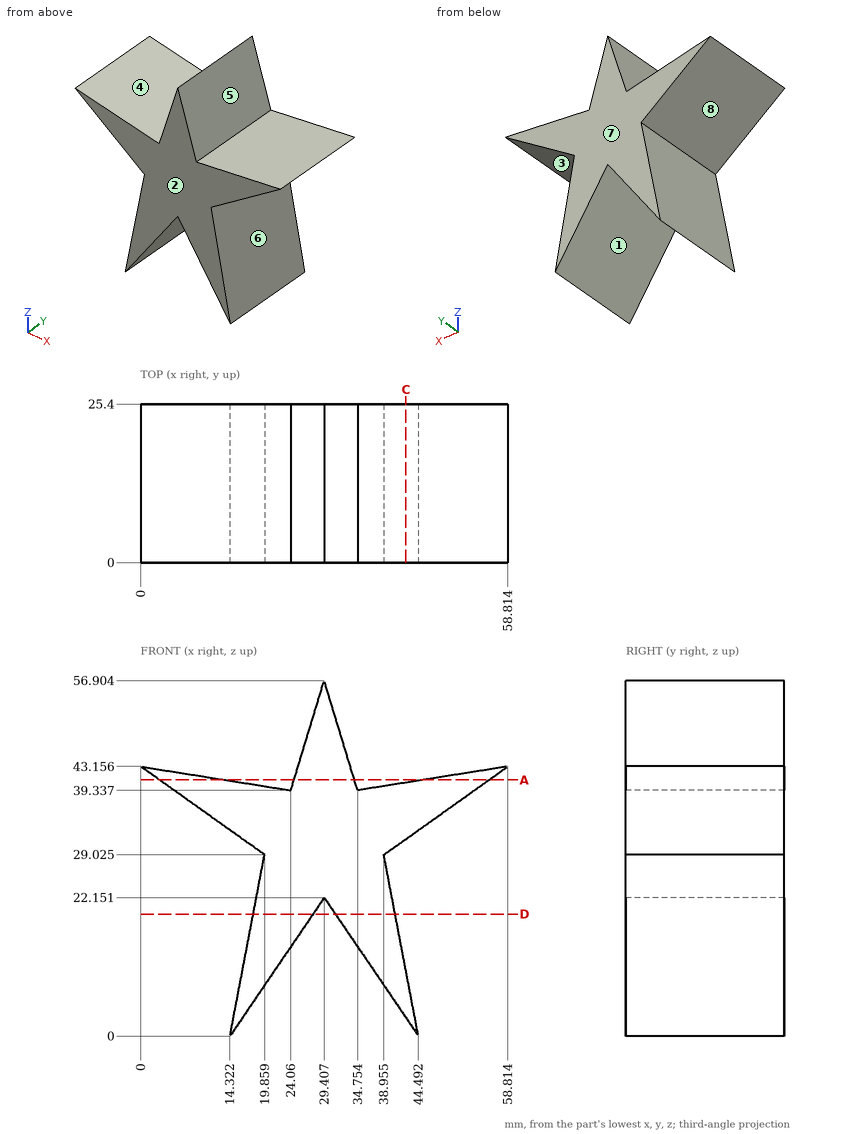
Input: dimensioned drawing with shaded views. Units: mm. Origin: part minimum x, y, z. A direction names the side the tool comes from. Coordinates: 2 decimals unless noted, no trailing zeros. Order: outer loops, then holes, each group sorted by start corner. A loop starts at its lowest first (then second) coordinate and runs counter-clockwise, first axis right, second up. Notation, with made-up numbers: (-12, 24) -> (8, 24) arc R28 cw to (8, 47) -> close; hole circle Ø10 at (36.25, 38). An arc over 180 degrees is marked (long way). Use CSV: the item, a comma, the result in double quotes.
1) Line query: line 1 (X direction, y = 24, z = 19) (1 decimal); line 2 (X direction, y = 22.5, z = 5.5) (1 decimal); line 3 (Z direction, x = 56, y = 22) (1 decimal). Output: solid intervals per line, ascending.
Findings:
line 1,"x = 17.9 to 27.3, 31.6 to 40.9"
line 2,"x = 15.4 to 18.1, 40.7 to 43.4"
line 3,"z = 41.2 to 42.7"
2) Mould query, pull axis Z, two halves, no side actions, for the marked faces 1, 2, 3 and 4. Classes: +Z half, -Z half, draft (parallel to the pull), parting line (faces both ways), or undercut.
Findings:
face 1,"-Z half"
face 2,"draft"
face 3,"undercut"
face 4,"+Z half"
3) Access query for the marked faces 5, 6, 7 and 8. Directions: +Z, -Z, +X, -X, +Y, -Y. A direction counts if a zero-diameter tool reaches every point of the face in a straight line with its end or side. Return the directions, or none.
Findings:
face 5,"+Z, +Y, -Y"
face 6,"+X, +Y, -Y"
face 7,"+Z, -Z, +X, -X, +Y"
face 8,"-X, +Y, -Y"
4) Pin query (flat end, axial travel): pin 1 Ø3 at (x, y) = (20, 2.5) entering from -Z (1 decimal); pin 2 Ø5 at (x, y) = (7.5, 18) entering from -Z; pin 3 Ø5 at (x, y) = (44, 18.5) entering from -Z; pin 4 Ø3 at (y, z) = (7, 29.5) entering from -X (1 decimal). Return the tip coordinate at first contact, or that it passes through.
Findings:
pin 1,"stops at z = 6.1"
pin 2,"stops at z = 36.04"
pin 3,"stops at z = 0"
pin 4,"stops at x = 17.1"
5) Section A-A on z = 41. Output: boundary loops of the cut face in (x, y) (1 decimal).
Findings:
outline,"(3, 0) -> (13.6, 0) -> (13.6, 25.4) -> (3, 25.4) -> close; (24.6, 0) -> (34.2, 0) -> (34.2, 25.4) -> (24.6, 25.4) -> close; (45.2, 0) -> (55.8, 0) -> (55.8, 25.4) -> (45.2, 25.4) -> close"
6) Section C-C on x = 42.5. Output: boundary loops of the cut face in (y, z) (1 decimal).
Findings:
outline,"(0, 2.9) -> (25.4, 2.9) -> (25.4, 10.4) -> (0, 10.4) -> close; (0, 31.5) -> (25.4, 31.5) -> (25.4, 40.6) -> (0, 40.6) -> close"
7) Section D-D on z = 19.5. Output: boundary loops of the cut face in (x, y).
Findings:
outline,"(18.04, 0) -> (27.6, 0) -> (27.6, 25.4) -> (18.04, 25.4) -> close; (31.21, 0) -> (40.77, 0) -> (40.77, 25.4) -> (31.21, 25.4) -> close"
